Work out the finished part from the listing and answer in its coordinate system (mm). Face numbers are marked on the shaded views. Coordinates: 2 decimals unless noted, no trailing zeros. Order: outer loops, then holes, each group sorted by start corner. A loop starts at its lowest first (then second) coordinate and runs counter-clockwise, first axis right, second up. Notation, with made-up numbers: M 39,84.5 L 52,84.5 A14 ccw 52,104.5 Z; hole C -15.75,39 d6. An arc over 180 degrees is marked long. Use a Markdown table: item, result.
from build123d import *


with BuildPart() as f1:
    # F0 (on Front) → F1 (revolve)
    with BuildSketch(Plane.XZ):
        Polygon((1.4, 14), (0.7, 14), (0.7, -14), (1.4, -14), (1.4, -9.5), (1.4, -5), (1.4, -0.5), (1.4, 0.5), (1.4, 3.744), (1.4, 6.308), (1.4, 8.872), (1.4, 11.436), align=None)
        Polygon((1.8, 11.5), (1.4, 14), (1.4, 11.436), align=None)
        Polygon((1.8, 8.936), (1.4, 11.436), (1.4, 8.872), align=None)
        Polygon((1.8, 6.372), (1.4, 8.872), (1.4, 6.308), align=None)
        Polygon((1.8, 3.808), (1.4, 6.308), (1.4, 3.744), align=None)
        Polygon((1.4, 0.5), (1.4, -0.5), (2.4, -0.5), align=None)
        Polygon((1.4, -0.5), (1.4, -5), (2.4, -0.5), align=None)
        Polygon((1.4, -5), (1.4, -9.5), (2.4, -5), align=None)
        Polygon((1.4, -9.5), (1.4, -14), (2.4, -9.5), align=None)
    revolve(axis=Axis((0, 0, 0.375825), (0, 0, -1)))


solid = f1.part
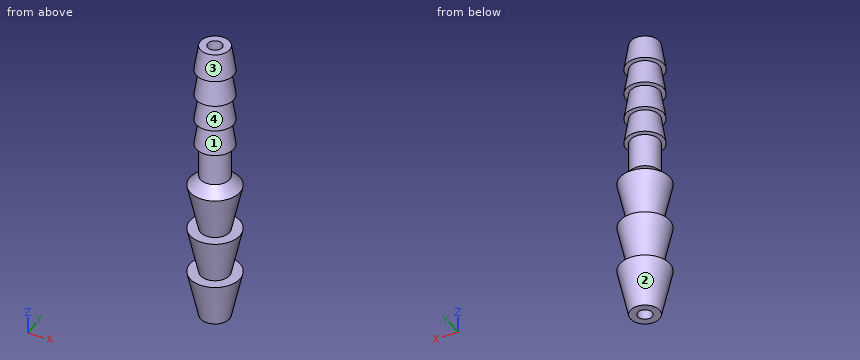
1. For a pull along Z with two mould halves and no side action, classify the marked faces 1, 2, 3 and 4 as +Z half, -Z half, draft (parallel to the pull), parting line (faces both ways), or undercut.
Answers below:
| item | result |
|---|---|
| face 1 | undercut |
| face 2 | -Z half |
| face 3 | +Z half |
| face 4 | undercut |
2. Flat-ended cylindrical pins translate along their axes: P1, Ø1.5, axis at x = 0, y = 0.5, coming from the +Z side; P2, Ø2, axis at x = -1.5, z = -3.5, coming from the -Y side; P3, Ø1, axis at x = -1, z = -8.5, coming from the +Y side; P4, Ø1.5, axis at y = 1, z = -5.5, coming from the +X side. Find the tip coordinate at first contact, or state that the pin passes through.
Answers below:
| item | result |
|---|---|
| P1 | z = 14 |
| P2 | y = -1.73 |
| P3 | y = 1.58 |
| P4 | x = 2.36 |
3. Section A-A on z = 3 is taken. Determine the outline of the cut face in (x, y).
Answers below:
| item | result |
|---|---|
| outline | C 0,0 d2.8; hole C 0,0 d1.4 |
4. Section C-C on z = -6.25 is taken. Determine the outline of the cut face in (x, y), then the cut area to 3 significant figures.
Answers below:
| item | result |
|---|---|
| outline | C 0,0 d4.24; hole C 0,0 d1.4 |
| area | 12.6 mm² |
5. Find the intervals of material crossed by probe 1 along Y at (x, z) = (0.4, 5.25); probe 2 along X at (y, z) = (0, 4.75); probe 3 along X at (y, z) = (0, -1.5), in increasing order.
Answers below:
| item | result |
|---|---|
| probe 1 | -1.52 to -0.57, 0.57 to 1.52 |
| probe 2 | -1.65 to -0.7, 0.7 to 1.65 |
| probe 3 | -2.18 to -0.7, 0.7 to 2.18 |
6. Section B-B on y = 2.05 is taken. Give the number of separate pieces and of enclosed holes in the cut face, then the cut area to 3 significant figures.
Answers below:
| item | result |
|---|---|
| separate pieces | 3 |
| enclosed holes | 0 |
| area | 8.31 mm² |
